The listing builds one solid part. Answer for the finished solid, in the listing's coordinates (mm). Face numbers are marked on the shaded views. A direction names the side the tool comes from. Round coordinates to 2 decimals unless told otherwise and drop trailing zeros. Order: outer loops, then holes, each group sorted by start corner. A loop starts at its lowest first (then second) coordinate and runs counter-clockwise, first axis right, second up. Notation, with made-up numbers: (44.25, -6.75) - (59.25, -6.75) arc R14 cw to (59.25, -0.75) - close; hole circle Ø8 at (37, 34.5). An arc over 180 degrees is marked (long way). One line per item, written item: value. Start each with the question number.
1. Straight lines are drawn through the part: line 1 (X direction, y = -70.5, z = 8.5); line 2 (X direction, y = -66.5, z = 10); line 3 (Z direction, x = 24, y = -49). For each, find the intervals that lie inside material, in ascending order.
2. Section D-D, the plane x = 5 is taken. Give the vertices of the cut face in (y, z).
3. Section B-B, the plane z = 3 is taken. Give the vertices of the cut face in (x, y), then the cut area to 3 significant figures.
4. A tool of negligible diameter and unlimited length cuts with its end or side. For the marked faces 1, 2 and 3, from which of +Z, -Z, +X, -X, +Y, -Y can it reach the whole face along a straight path? Write none if from no direction.
5. A flat-ended cylindrical pin translates along its axis: P1, Ø6, axis at y = -34, z = 44, coming from the +X side. Find the tip coordinate at first contact, or state that the pin passes through.
6. For a pull along X with two mould halves and no side action, classify the marked faces 4, 5, 6 and 7 as released by +X, released by -X, zero draft, split by the parting line, or undercut.
7. Section A-A, the plane y = -69.5 is taken. Give the vertices of the cut face in (x, z), then the cut area to 3 significant figures.
8. Section C-C, the plane y = -38 is taken. Give the vertices of the cut face in (x, z).
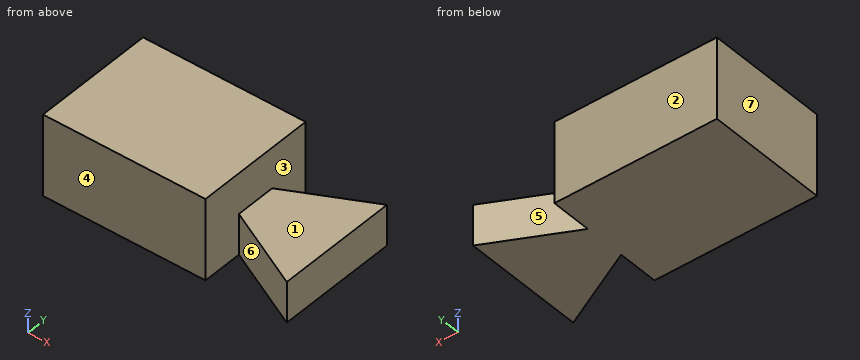
from build123d import *

# Parameters (mm, degrees)
F0_W     = 101.6
F0_H     = 50.8
F1_DEPTH = 76.2
F3_DEPTH = 25.4


with BuildPart() as f1:
    # F0 (on Front) → F1 (new body)
    with BuildSketch(Plane.XZ):
        with Locations((-50.8, 25.4)):
            Rectangle(F0_W, F0_H)
    extrude(amount=F1_DEPTH)

    # F2 (on face) → F3 (join)
    with BuildSketch(Plane(origin=(0, 0, 0), x_dir=(1, 0, 0), z_dir=(0, 0, -1))):
        Polygon((0, 50.8), (0, 25.4), (50.9050786495, 0), (50.8, 76.2), align=None)
    extrude(amount=-F3_DEPTH)


solid = f1.part
Answer list:
1. line 1: x = -101.6 to 0, 39.4 to 50.81
1. line 2: x = -101.6 to 0, 31.4 to 50.81
1. line 3: z = 0 to 25.4
2. outline: (-53.3, 0) - (-22.91, 0) - (-22.91, 25.4) - (-53.3, 25.4) - close
3. outline: (-101.6, -76.2) - (0, -76.2) - (0, -50.8) - (50.8, -76.2) - (50.91, 0) - (0, -25.4) - (0, 0) - (-101.6, 0) - close
3. area: 10,300 mm²
4. face 1: +Z, +X, +Y, -Y
4. face 2: +Z, -Z, +X, -X, +Y
4. face 3: +Z
5. P1: stops at x = 0
6. face 4: zero draft
6. face 5: undercut
6. face 6: undercut
6. face 7: released by -X
7. outline: (-101.6, 0) - (0, 0) - (0, 50.8) - (-101.6, 50.8) - close; (37.4, 0) - (50.81, 0) - (50.81, 25.4) - (37.4, 25.4) - close
7. area: 5,500 mm²
8. outline: (-101.6, 0) - (50.85, 0) - (50.85, 25.4) - (0, 25.4) - (0, 50.8) - (-101.6, 50.8) - close
